Read the model definition and answer for the solid it produces. Units are mm, in the model's axes. A direction names the side the tool comes from. Give positions to 0.01 mm unless a question says otherwise; leave off trailing zeros. Order: outer loops, then holes, each group sorted by start corner. A loop starts at its lowest first (then second) coordinate and runs counter-clockwise, first axis right, second up.
```python
from build123d import *

# Parameters (mm, degrees)
SKETCH1_W           = 200
SKETCH1_H           = 160
BOSS_EXTRUDE1_DEPTH = 5
SKETCH2_R           = 2
CUT_EXTRUDE1_DEPTH  = 5
SKETCH3_R           = 1.5
CUT_EXTRUDE4_DEPTH  = 5
SKETCH4_R           = 1.5
CUT_EXTRUDE5_DEPTH  = 5
SKETCH5_W           = 35
SKETCH5_H           = 35
CUT_EXTRUDE6_DEPTH  = 5
SKETCH7_W           = 7
SKETCH7_H           = 40
SKETCH7_W_2         = 5
SKETCH7_W_3         = 20
SKETCH7_H_2         = 5
CUT_EXTRUDE7_DEPTH  = 5
SKETCH8_W           = 15
SKETCH8_H           = 12
SKETCH8_W_2         = 30
SKETCH8_H_2         = 6
CUT_EXTRUDE8_DEPTH  = 5
SKETCH9_W           = 20
SKETCH9_H           = 5
CUT_EXTRUDE9_DEPTH  = 5
SKETCH10_R          = 1.5
CUT_EXTRUDE10_DEPTH = 5
SKETCH11_R          = 1.5
CUT_EXTRUDE11_DEPTH = 5
SKETCH12_R          = 1.5
CUT_EXTRUDE12_DEPTH = 5


with BuildPart() as part:
    # Sketch1 → Boss-Extrude1 (new body)
    with BuildSketch(Plane(origin=(0, 0, 0), x_dir=(1, 0, 0), z_dir=(0, 1, 0))):
        Rectangle(SKETCH1_W, SKETCH1_H)
    extrude(amount=BOSS_EXTRUDE1_DEPTH)

    # Sketch2 → Cut-Extrude1 (cut)
    with BuildSketch(Plane(origin=(0, 5, 0), x_dir=(1, 0, 0), z_dir=(0, 1, 0))):
        with Locations(Location((-93, 73, 0), (0, 0, 270))):
            Circle(SKETCH2_R)
        with Locations(Location((93, 73, 0), (0, 0, 90))):
            Circle(SKETCH2_R)
        with Locations(Location((93, -73, 0), (0, 0, 270))):
            Circle(SKETCH2_R)
        with Locations(Location((-93, -73, 0), (0, 0, 90))):
            Circle(SKETCH2_R)
    extrude(amount=-CUT_EXTRUDE1_DEPTH, mode=Mode.SUBTRACT)

    # Sketch3 → Cut-Extrude4 (cut)
    with BuildSketch(Plane(origin=(0, 5, 0), x_dir=(1, 0, 0), z_dir=(0, 1, 0))):
        with Locations(Location((90, 7.5, 0), (0, 0, 270))):
            Circle(SKETCH3_R)
        with Locations(Location((90, -7.5, 0), (0, 0, 90))):
            Circle(SKETCH3_R)
    extrude(amount=-CUT_EXTRUDE4_DEPTH, mode=Mode.SUBTRACT)

    # Sketch4 → Cut-Extrude5 (cut)
    with BuildSketch(Plane(origin=(0, 5, 0), x_dir=(1, 0, 0), z_dir=(0, 1, 0))):
        with Locations(Location((55, 36, 0), (0, 0, 270))):
            Circle(SKETCH4_R)
        with Locations(Location((55, -36, 0), (0, 0, 90))):
            Circle(SKETCH4_R)
    extrude(amount=-CUT_EXTRUDE5_DEPTH, mode=Mode.SUBTRACT)

    # Sketch5 → Cut-Extrude6 (cut)
    with BuildSketch(Plane(origin=(0, 5, 0), x_dir=(1, 0, 0), z_dir=(0, 1, 0))):
        with Locations((2.5, 0)):
            Rectangle(SKETCH5_W, SKETCH5_H)
    extrude(amount=-CUT_EXTRUDE6_DEPTH, mode=Mode.SUBTRACT)

    # Sketch7 → Cut-Extrude7 (cut)
    with BuildSketch(Plane(origin=(0, 5, 0), x_dir=(1, 0, 0), z_dir=(0, 1, 0))):
        with Locations((-11.5, -50)):
            Rectangle(SKETCH7_W, SKETCH7_H)
        with Locations((32.5, 0)):
            Rectangle(SKETCH7_W_2, SKETCH7_H)
        with Locations((-30, 67.5)):
            Rectangle(SKETCH7_W_3, SKETCH7_H_2)
        with Locations((-30, -67.5)):
            Rectangle(SKETCH7_W_3, SKETCH7_H_2)
    extrude(amount=-CUT_EXTRUDE7_DEPTH, mode=Mode.SUBTRACT)

    # Sketch8 → Cut-Extrude8 (cut)
    with BuildSketch(Plane(origin=(0, 5, 0), x_dir=(1, 0, 0), z_dir=(0, 1, 0))):
        with Locations((17.5, 28.5)):
            Rectangle(SKETCH8_W, SKETCH8_H)
        with Locations((85, 43)):
            Rectangle(SKETCH8_W_2, SKETCH8_H_2)
        with Locations((85, -43)):
            Rectangle(SKETCH8_W_2, SKETCH8_H_2)
    extrude(amount=-CUT_EXTRUDE8_DEPTH, mode=Mode.SUBTRACT)

    # Sketch9 → Cut-Extrude9 (cut)
    with BuildSketch(Plane(origin=(0, 5, 0), x_dir=(1, 0, 0), z_dir=(0, 1, 0))):
        with Locations((20, 67.5)):
            Rectangle(SKETCH9_W, SKETCH9_H)
    extrude(amount=-CUT_EXTRUDE9_DEPTH, mode=Mode.SUBTRACT)

    # Sketch10 → Cut-Extrude10 (cut)
    with BuildSketch(Plane(origin=(0, 5, 0), x_dir=(1, 0, 0), z_dir=(0, 1, 0))):
        with Locations(Location((-95, -25, 0), (0, 0, 270))):
            Circle(SKETCH10_R)
        with Locations(Location((-45, 68, 0), (0, 0, 270))):
            Circle(SKETCH10_R)
    extrude(amount=-CUT_EXTRUDE10_DEPTH, mode=Mode.SUBTRACT)

    # Sketch11 → Cut-Extrude11 (cut)
    with BuildSketch(Plane(origin=(0, 5, 0), x_dir=(1, 0, 0), z_dir=(0, 1, 0))):
        with Locations(Location((2, -33, 0), (0, 0, 270))):
            Circle(SKETCH11_R)
        with Locations(Location((2, -70, 0), (0, 0, 90))):
            Circle(SKETCH11_R)
        with Locations(Location((39, -70, 0), (0, 0, 270))):
            Circle(SKETCH11_R)
        with Locations(Location((39, -33, 0), (0, 0, 90))):
            Circle(SKETCH11_R)
    extrude(amount=-CUT_EXTRUDE11_DEPTH, mode=Mode.SUBTRACT)

    # Sketch12 → Cut-Extrude12 (cut)
    with BuildSketch(Plane(origin=(0, 5, 0), x_dir=(1, 0, 0), z_dir=(0, 1, 0))):
        with Locations(Location((-65, 55, 0), (0, 0, 270))):
            Circle(SKETCH12_R)
        with Locations(Location((-65, -55, 0), (0, 0, 90))):
            Circle(SKETCH12_R)
    extrude(amount=-CUT_EXTRUDE12_DEPTH, mode=Mode.SUBTRACT)


solid = part.part
```
1) The part is cut by section A-A on x = -26. Determine the outline of the cut face in (y, z).
Final values:
outline: (0, -80) - (5, -80) - (5, -70) - (0, -70) - close; (0, -65) - (5, -65) - (5, 65) - (0, 65) - close; (0, 70) - (5, 70) - (5, 80) - (0, 80) - close
2) A tool of negligible diameter and unlimited length cuts with its end or side. For faces 1 (the face through (70, 3, 43)), 2 (the face through (-8, 3, 50)), 3 (the face through (-100, 2, 1)), from which of +Z, -Z, +X, -X, +Y, -Y can it reach the whole face along a straight path? Write none if from no direction.
Final values:
face 1: +X, +Y, -Y
face 2: +Y, -Y
face 3: +Z, -Z, -X, +Y, -Y
3) For a pull along Z with two mould halves and no side action, classify faces 4 (the face through (10, 3, -28)), 5 (the face through (-1, 2, 80)), 6 (the face through (100, 2, -63)) as released by +Z, released by -Z, zero draft, split by the parting line, or undercut.
Final values:
face 4: undercut
face 5: released by +Z
face 6: zero draft
4) The part is cut by section B-B on z = 0. Determine the outline of the cut face in (x, y), and give its area (3 significant figures).
Final values:
outline: (-100, 0) - (-15, 0) - (-15, 5) - (-100, 5) - close; (20, 0) - (30, 0) - (30, 5) - (20, 5) - close; (35, 0) - (100, 0) - (100, 5) - (35, 5) - close
area: 800 mm2
5) Consider L1, parallel to X at y = 3.8, z = -73; L2, parallel to X at y = 1.55, z = 7.5; L3, parallel to X at y = 4.5, z = 16. Determine where each line is inside the solid, lowest interval first.
Final values:
L1: x = -100 to -95, -91 to 91, 95 to 100
L2: x = -100 to -15, 20 to 30, 35 to 88.5, 91.5 to 100
L3: x = -100 to -15, 20 to 30, 35 to 100
